Geometry: final body of the model. Coordinates: model frame, mm. A direction names the side the tool comes from. Coordinates: 2 decimals unless noted, no trailing zeros. Loops run counter-clockwise (first coordinate to the right, second up) from the corner with the lowest first, then second, coordinate; pieces in that order, holes last. Notation, with made-up numbers: (5, 63) - (59, 63) arc R30 cw to (59, 91) - close; hole circle Ø7 at (83.25, -19.75). An arc over 180 degrees is marked (long way). Put each result on its own line as item: value. Start each with the question number.
1) Material intervals for line 1 along X through (y, z) = (1.75, 18); line 2 along Y through (x, z) = (3.25, 2.5); line 3 along Z through (x, y) = (-2.5, 1), sorted ascending. Write a range as from..to.
2) Contact query for flat-ended pins moving along their axis: pin 1 Ø6 at (x, z) = (-4, 0) entering from +Y; pin 2 Ø0.8 at (x, y) = (5.5, -1) entering from -Z; pin 3 Ø4 at (x, z) = (2.5, 11) entering from -Y. Output: stop coordinate, or through.
3) Draft query along X for faces 5 (the flat face through (-5.08, 1, 15)), 6 (the flat face through (5.6, -1, 13.462)), 7 (the flat face through (6.096, 1, 6)). Return one class per face: +X half, -X half, draft (parallel to the pull), parting line (faces both ways), or undercut.
4) Reachability of faces 1 (the flat face through (0, 1, 13.462)), 2 (the flat face through (-6.096, 1, 6)), 3 (the flat face through (-5.6, 3, 13.462)), 4 (the flat face through (-5.6, -1, 13.462)) from +Z, -Z, +X, -X, +Y, -Y: full face, straight path, thin tool, end or side. Return the list, or none.
5) Section B-B on y = 3.25. Output: boundary loops of the cut face in (x, z), and give its area (3 significant figures).
6) Section D-D on z = -11. Output: boundary loops of the cut face in (x, y).
7) Section C-C on x = -0.5. Output: boundary loops of the cut face in (y, z).
8) Section A-A on y = 1. Output: boundary loops of the cut face in (x, z) (3 decimals), and give its area (3 significant figures).
```python
from build123d import *

# Parameters (mm, degrees)
SKETCH1_W               = 12.192
SKETCH1_H               = 30.734
BOSS_EXTRUDE1_DEPTH     = 2
BOSS_EXTRUDE2_DEPTH     = 12.192
SKETCH3_R               = 1.25
CUT_EXTRUDE1_DEPTH      = 24.505965051
CUT_EXTRUDE2_DEPTH      = 22.001112947
CUT_EXTRUDE2_DEPTH_BACK = 22.001112947
SKETCH4_W               = 10.16
SKETCH4_H               = 6.223


with BuildPart() as part:
    # Sketch1 → Boss-Extrude1 (new body)
    with BuildSketch(Plane(origin=(0, 0, 0), x_dir=(1, 0, 0), z_dir=(0, 1, 0))):
        Rectangle(SKETCH1_W, SKETCH1_H)
    extrude(amount=BOSS_EXTRUDE1_DEPTH)

    # Sketch2 → Boss-Extrude2 (add)
    with BuildSketch(Plane(origin=(6.096, 0, 0), x_dir=(0, 0, -1), z_dir=(1, 0, 0))):
        with BuildLine():
            ThreePointArc((-13.757711199, 0), (-14.618095322, -1.28349029), (-15.997337956, -1.980123566))
            Line((-15.997337956, -1.980123566), (-13.462, -2.048))
            Line((-13.462, -2.048), (-13.462, 0))
            Line((-13.462, 0), (-13.757711199, 0))
        make_face()
        with BuildLine():
            Line((-13.462, 2), (-13.757711199, 2))
            ThreePointArc((-13.757711199, 2), (-13.631473734, 1.50706594), (-13.589, 1))
            ThreePointArc((-13.589, 1), (-13.631473734, 0.49293406), (-13.757711199, 0))
            Line((-13.757711199, 0), (-13.462, 0))
            Line((-13.462, 0), (-13.462, 2))
        make_face()
        with BuildLine():
            Line((-13.462, 4.048), (-16.637, 4.048))
            ThreePointArc((-16.637, 4.048), (-14.870321761, 3.483777768), (-13.757711199, 2))
            Line((-13.757711199, 2), (-13.462, 2))
            Line((-13.462, 2), (-13.462, 4.048))
        make_face()
        with BuildLine():
            ThreePointArc((-13.757711199, 2), (-14.870321761, 3.483777768), (-16.637, 4.048))
            ThreePointArc((-16.637, 4.048), (-19.658290199, 1.402628284), (-17.435200057, -1.941628914))
            Line((-17.435200057, -1.941628914), (-15.997337956, -1.980123566))
            ThreePointArc((-15.997337956, -1.980123566), (-14.618095322, -1.28349029), (-13.757711199, 0))
            Line((-13.757711199, 0), (-15.367, 0))
            Line((-15.367, 0), (-15.367, 2))
            Line((-15.367, 2), (-13.757711199, 2))
        make_face()
    extrude(amount=-BOSS_EXTRUDE2_DEPTH)

    # Sketch3 → Cut-Extrude1 (cut, through all)
    with BuildSketch(Plane(origin=(6.096, 0, 0), x_dir=(0, 0, -1), z_dir=(1, 0, 0))):
        with Locations((-16.637, 1)):
            Circle(SKETCH3_R)
    extrude(amount=-CUT_EXTRUDE1_DEPTH, mode=Mode.SUBTRACT)

    # Sketch4 → Cut-Extrude2 (cut, two sides: drawn at the far end of the back side and taken through both)
    with BuildSketch(Plane(origin=(0, 2, 0), x_dir=(1, 0, 0), z_dir=(0, 1, 0)).offset(-CUT_EXTRUDE2_DEPTH_BACK)):
        with Locations((0, -16.5735)):
            Rectangle(SKETCH4_W, SKETCH4_H)
    extrude(amount=CUT_EXTRUDE2_DEPTH + CUT_EXTRUDE2_DEPTH_BACK, mode=Mode.SUBTRACT)


solid = part.part
```
Answer block:
1. line 1: x = -6.1..-5.08, 5.08..6.1
1. line 2: y = 0..2
1. line 3: z = -15.37..13.46
2. pin 1: stops at y = 2
2. pin 2: stops at z = 13.46
2. pin 3: stops at y = 0
3. face 5: undercut
3. face 6: draft
3. face 7: +X half
4. face 1: +Z, +Y, -Y
4. face 2: +Z, -Z, -X, +Y, -Y
4. face 3: -Z, +X, -X, +Y
4. face 4: -Z, +X, -X, -Y
5. outline: (-6.1, 13.46) - (-5.08, 13.46) - (-5.08, 18.69) - (-6.1, 18.69) - close; (5.08, 13.46) - (6.1, 13.46) - (6.1, 18.69) - (5.08, 18.69) - close
5. area: 10.6 mm²
6. outline: (-6.1, 0) - (6.1, 0) - (6.1, 2) - (-6.1, 2) - close
7. outline: (0, -15.37) - (2, -15.37) - (2, 13.46) - (0, 13.46) - close
8. outline: (-6.096, -15.367) - (6.096, -15.367) - (6.096, 15.387) - (5.08, 15.387) - (5.08, 13.462) - (-5.08, 13.462) - (-5.08, 15.387) - (-6.096, 15.387) - close; (-6.096, 17.887) - (-5.08, 17.887) - (-5.08, 19.685) - (-6.096, 19.685) - close; (5.08, 17.887) - (6.096, 17.887) - (6.096, 19.685) - (5.08, 19.685) - close
8. area: 359 mm²
